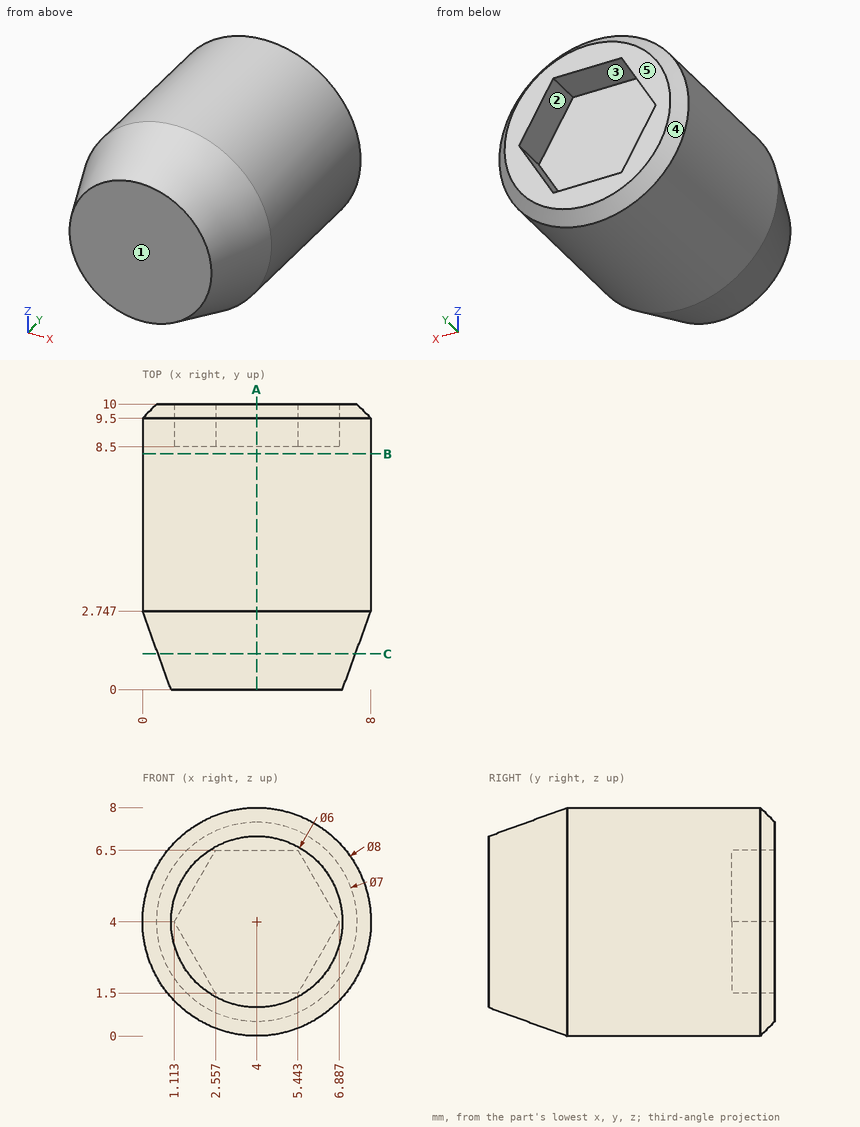
Study the drawing (mm; zero at the part's minimum x, y, z) and answer. A direction names the side the tool comes from. Coordinates: 2 decimals unless noted, no trailing zeros. Order: outer loops, then holes, each group sorted by start corner. A loop starts at its lowest first (then second) coordinate and runs counter-clockwise, first axis right, second up. Notation, with made-up numbers: M 53.25,-24.5 L 101.25,-24.5 A11 ccw 101.25,-4.5 Z; hole C 55.25,68.25 d1. An arc over 180 degrees is marked long. Answer as a JSON object with one key per item and string values. Group by question number.
1. Section A-A on x = 4 is taken. Write down the section's boundary in (y, z).
2. A tool of negligible diameter and unlimited length cuts with its end or side. For the marked faces 1 and 2, from which of +Z, -Z, +X, -X, +Y, -Y can it reach the whole face along a straight path? Write none if from no direction.
3. Section C-C on y = 1.25 is taken. Write down the section's boundary in (x, z) (1 decimal), then the cut area to 3 significant figures.
4. Determine the mould class of the marked faces 3, 4 and 5 for opening direction Z: released by +Z, released by -Z, zero draft, split by the parting line, or undercut.
5. Flat-ended cylindrical pins translate along their axes: P1, Ø2, axis at y = 3.5, z = 5.5, coming from the -X side; P2, Ø2.5, axis at x = 3, z = 4, coming from the +Y side; P3, Ø4, axis at y = 3.5, z = 1, coming from the -X side. Find the tip coordinate at first contact, or state that the pin passes through.
6. Section B-B on y = 8.25 is taken. Write down the section's boundary in (x, z).
7. Straight lines are drawn through the part: line 1 (Y direction, x = 4.25, z = 5.5); line 2 (X direction, y = 8.75, z = 2.75) (1 decimal); line 3 (Z direction, x = 1, y = 7.5) (1 decimal). For each, find the intervals that lie inside material, in ascending order.
Values follow:
{
 "1": {"outline": "M 0,1 L 2.75,0 L 9.5,0 L 10,0.5 L 10,1.5 L 8.5,1.5 L 8.5,6.5 L 10,6.5 L 10,7.5 L 9.5,8 L 2.75,8 L 0,7 Z"},
 "2": {"face 1": "+Z, -Z, +X, -X, -Y", "face 2": "+Y"},
 "3": {"outline": "C 4,4 d6.9", "area": "37.5 mm2"},
 "4": {"face 3": "undercut", "face 4": "split by the parting line", "face 5": "zero draft"},
 "5": {"P1": "x = 0.03", "P2": "y = 8.5", "P3": "x = 0.13"},
 "6": {"outline": "C 4,4 d8"},
 "7": {"line 1": "0 to 8.5", "line 2": "0.2 to 1.8, 6.2 to 7.8", "line 3": "1.4 to 6.6"}
}
